CAD build for the part. Positions are in the model's coordinates, mm. Face numbers are marked on the shaded views. A direction names the side the tool comes from. Give positions to 0.01 mm unless a question says otherwise; leave off trailing zeros. Write each loop counter-clockwise with the first axis right and the second up, starting at its lowest first coordinate (ties: lowest second). Pieces come first, ordered by that corner, then holes. Notation, with made-up numbers: (6, 13) -> (43, 13) arc R17 ccw to (43, 22) -> close; hole circle Ø5 at (-14, 62.5). An arc over 180 degrees is marked (long way). Use one line per item in the form item = value. Start each with the question number.
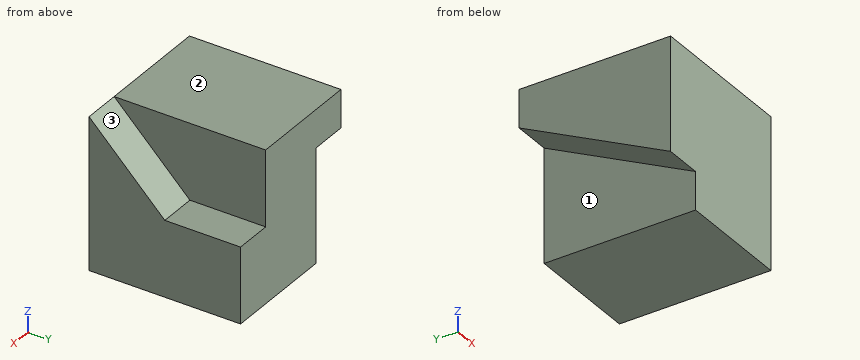
from build123d import *

# Parameters (mm, degrees)
SKETCH1_W           = 40
SKETCH1_H           = 40
BOSS_EXTRUDE1_DEPTH = 40
SKETCH2_W           = 10
SKETCH2_H           = 10
CUT_EXTRUDE1_DEPTH  = 40
SKETCH6_W           = 10
SKETCH6_H           = 20
CUT_EXTRUDE4_DEPTH  = 20
SKETCH7_W           = 10
SKETCH7_H           = 20
CUT_EXTRUDE5_DEPTH  = 10
SKETCH12_W          = 10
SKETCH12_H          = 20
CUT_EXTRUDE11_DEPTH = 10
SKETCH13_W          = 10
SKETCH13_H          = 20
BOSS_EXTRUDE4_DEPTH = 10
CUT_EXTRUDE12_DEPTH = 10
BOSS_EXTRUDE5_DEPTH = 10
CUT_EXTRUDE15_DEPTH = 10


with BuildPart() as part:
    # Sketch1 → Boss-Extrude1 (new body)
    with BuildSketch(Plane.XY):
        with Locations((20, 20)):
            Rectangle(SKETCH1_W, SKETCH1_H)
    extrude(amount=BOSS_EXTRUDE1_DEPTH)

    # Sketch2 → Cut-Extrude1 (cut)
    with BuildSketch(Plane(origin=(0, 40, 0), x_dir=(1, 0, 0), z_dir=(0, 1, 0))):
        with Locations((5, -5)):
            Rectangle(SKETCH2_W, SKETCH2_H)
    extrude(amount=-CUT_EXTRUDE1_DEPTH, mode=Mode.SUBTRACT)

    # Sketch6 → Cut-Extrude4 (cut)
    with BuildSketch(Plane.XY.offset(40)):
        with Locations((35, 30)):
            Rectangle(SKETCH6_W, SKETCH6_H)
    extrude(amount=-CUT_EXTRUDE4_DEPTH, mode=Mode.SUBTRACT)

    # Sketch7 → Cut-Extrude5 (cut)
    with BuildSketch(Plane.XY.offset(40)):
        with Locations((35, 10)):
            Rectangle(SKETCH7_W, SKETCH7_H)
    extrude(amount=-CUT_EXTRUDE5_DEPTH, mode=Mode.SUBTRACT)

    # Sketch12 → Cut-Extrude11 (cut)
    with BuildSketch(Plane(origin=(0, 40, 0), x_dir=(1, 0, 0), z_dir=(0, 1, 0))):
        with Locations((5, -20)):
            Rectangle(SKETCH12_W, SKETCH12_H)
    extrude(amount=-CUT_EXTRUDE11_DEPTH, mode=Mode.SUBTRACT)

    # Sketch13 → Boss-Extrude4 (add)
    with BuildSketch(Plane.XY.offset(30)):
        with Locations((35, 10)):
            Rectangle(SKETCH13_W, SKETCH13_H)
    extrude(amount=BOSS_EXTRUDE4_DEPTH)

    # Sketch15 → Cut-Extrude12 (cut)
    with BuildSketch(Plane(origin=(40, 0, 0), x_dir=(0, 0, -1), z_dir=(1, 0, 0))):
        Polygon((-20, 20), (-40, 0), (-40, 20), align=None)
    extrude(amount=-CUT_EXTRUDE12_DEPTH, mode=Mode.SUBTRACT)

    # Sketch16 → Boss-Extrude5 (add)
    with BuildSketch(Plane.ZY):
        Polygon((30, 40), (25, 30), (30, 30), align=None)
    extrude(amount=-BOSS_EXTRUDE5_DEPTH)

    # Sketch17 → Cut-Extrude15 (cut)
    with BuildSketch(Plane.ZY):
        Polygon((25, 30), (10, 0), (10, 30), align=None)
    extrude(amount=-CUT_EXTRUDE15_DEPTH, mode=Mode.SUBTRACT)


solid = part.part
1) Cut at C-C (y = 31). Give the cut face in (x, z).
2) Cut at A-A (y = 14). Give the cut face in (x, z).
3) Cut at B-B (z = 34). Give the cut face in (x, y).
4) 3-axis set-ups, long thin cutter, end or side, ignore diameter. For the marked faces 1, 2 and 3: which of +Z, -Z, +X, -X, +Y, -Y reach the whole face in a straight line?
5) Pin check, flat tips, straight feed: pin 1 (4 mm diameter, centred on x = 19, z = 9, fed in from -Y); pin 2 (8 mm diameter, centred on x = 36, y = 26, fed in from +Z); pin 3 (6 mm diameter, centred on y = 26.5, z = 32, fed in from +X). Stop position of each tip, or through.
6) Wall check: line 1 along X through (y, z) = (21, 25); line 2 along X through (y, z) = (35.5, 12.5); line 3 along Z through (x, y) = (33.5, 22). Give the ranges that are in metal, low to high. Write a range as from..to.
7) Cut at D-D (x = 7.5). Give the cut face in (y, z), and give its area (3 significant figures).
Final values:
q1.outline = (0, 25.5) -> (10, 25.5) -> (10, 0) -> (40, 0) -> (40, 20) -> (30, 20) -> (30, 40) -> (0, 40) -> close
q2.outline = (0, 17) -> (10, 17) -> (10, 0) -> (40, 0) -> (40, 26) -> (30, 26) -> (30, 40) -> (0, 40) -> close
q3.outline = (0, 0) -> (40, 0) -> (40, 6) -> (30, 6) -> (30, 40) -> (0, 40) -> close
q4.face_1 = -Z, -X, +Y
q4.face_2 = +Z, +X, -X, +Y, -Y
q4.face_3 = +Z, +X, +Y
q5.pin_1 = 0
q5.pin_2 = 20
q5.pin_3 = 30
q6.line_1 = 0..30
q6.line_2 = 10..40
q6.line_3 = 0..20
q7.outline = (0, 10) -> (40, 30) -> (40, 40) -> (0, 40) -> close
q7.area = 800 mm^2
